from build123d import *

# Parameters (mm, degrees)
SKETCH1_R                           = 18.923
BOSS_EXTRUDE1_DEPTH                 = 74.041
FILLET1_R                           = 0.508
CHAMFER1_SIZE                       = 1.016
CHAMFER1_SIZE2                      = 1.625939882
SKETCH4_R                           = 14.859
CUT_EXTRUDE1_DEPTH                  = 12.7
CHAMFER2_SIZE                       = 0.762
F_1_1_4_12_TAPPED_HOLE1_D           = 29.76626
F_1_1_4_12_TAPPED_HOLE1_DEPTH       = 61.341
F_1_1_4_12_TAPPED_HOLE1_CSINK_D     = 33.7058
F_1_1_4_12_TAPPED_HOLE1_CSINK_ANGLE = 90


with BuildPart() as part:
    # Sketch1 → Boss-Extrude1 (new body)
    with BuildSketch(Plane.XY):
        Circle(SKETCH1_R)
    extrude(amount=BOSS_EXTRUDE1_DEPTH)

    # Sketch3 → Revolve1 (revolve)
    with BuildSketch(Plane(origin=(0, 0, 0), x_dir=(1, 0, 0), z_dir=(0, 1, 0))):
        Polygon((0, -74.041), (22.098, -74.041), (22.098, -61.341), (18.923, -58.039), (0, -58.039), align=None)
    revolve(axis=Axis((0, 0, 0), (0, 0, 1)))

    # Fillet1
    fillet1_edges = [part.edges().sort_by_distance(p)[0] for p in [
        (-18.923, 0, 58.039),
        (-22.098, 0, 74.041),
        (-22.098, 0, 61.341),
    ]]
    fillet(fillet1_edges, radius=FILLET1_R)

    # Chamfer1
    chamfer1_edges = [part.edges().sort_by_distance(p)[0] for p in [
        (-18.923, 0, 0),
    ]]
    chamfer1_side = [part.faces().sort_by_distance(p)[0] for p in [
        (0, 0, 0),
    ]]
    chamfer(chamfer1_edges, length=CHAMFER1_SIZE, length2=CHAMFER1_SIZE2, reference=chamfer1_side[0])

    # Sketch4 → Cut-Extrude1 (cut)
    with BuildSketch(Plane(origin=(0, 0, 0), x_dir=(-1, 0, 0), z_dir=(0, 0, -1))):
        Circle(SKETCH4_R)
    extrude(amount=-CUT_EXTRUDE1_DEPTH, mode=Mode.SUBTRACT)

    # Chamfer2
    chamfer2_edges = [part.edges().sort_by_distance(p)[0] for p in [
        (14.859, 0, 0),
    ]]
    chamfer(chamfer2_edges, length=CHAMFER2_SIZE)

    # 1-1/4-12 Tapped Hole1
    with Locations(Plane.XY.offset(74.041)):
        with Locations((0, 0)):
            CounterSinkHole(F_1_1_4_12_TAPPED_HOLE1_D / 2, F_1_1_4_12_TAPPED_HOLE1_CSINK_D / 2, depth=F_1_1_4_12_TAPPED_HOLE1_DEPTH, counter_sink_angle=F_1_1_4_12_TAPPED_HOLE1_CSINK_ANGLE)


solid = part.part
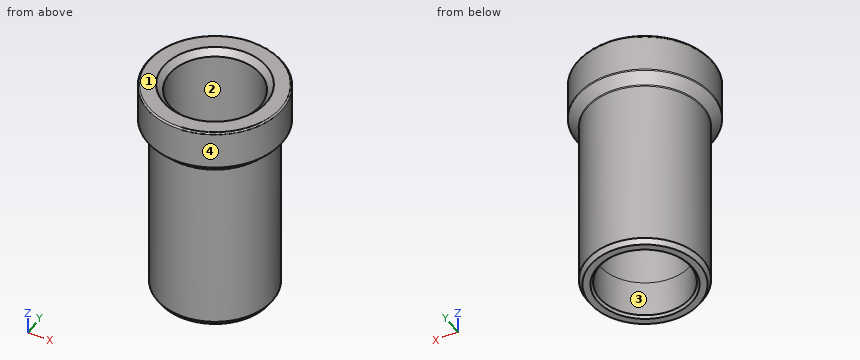
Read the model definition and answer for the solid it produces. Units are mm, in the model's axes. Face numbers are marked on the shaded views. Round coordinates to 2 decimals unless told otherwise and drop trailing zeros. Loops run counter-clockwise (first coordinate to the right, second up) from the corner with the lowest first, then second, coordinate; pieces in that order, holes last.
Q1. Consider probe 1 along Y at (x, z) = (0, 6); probe 2 along X at (y, z) = (0, 53); probe 3 along Y at (x, z) = (-3, 41). Determine where each line is inside the solid, lowest interval first.
Q2. Section A-A on z = 23.5 is taken. Write down the section's boundary in (x, y), and give its area (3 significant figures).
Q3. Each of these flat-tipped pins is pushed along its axis until it touches: pin 1 (12 mm diameter, centred on y = -11, z = 28, fed in from -X); pin 2 (4 mm diameter, centred on x = 5.5, z = 30, fed in from -Y); pin 3 (2 mm diameter, centred on y = -3, z = 23.5, fed in from -X). Where does it stop, or does it pass through?
Q4. Determine the mould class of the marked faces 1, 2, 3 and 4 for opening direction X: released by +X, released by -X, zero draft, split by the parting line, or undercut.
Output:
1. probe 1: y = -18.92 to -14.86, 14.86 to 18.92
1. probe 2: x = -18.92 to -14.88, 14.88 to 18.92
1. probe 3: y = -18.68 to -14.58, 14.58 to 18.68
2. outline: circle Ø37.85 at (0, 0); hole circle Ø29.77 at (0, 0)
2. area: 429 mm2
3. pin 1: stops at x = -18.25
3. pin 2: stops at y = -18.6
3. pin 3: stops at x = -18.82
4. face 1: zero draft
4. face 2: undercut
4. face 3: undercut
4. face 4: split by the parting line
